Read the model definition and answer for the solid it produces. Units are mm, in the model's axes. Face numbers are marked on the shaded views. A direction names the side the tool comes from. Round coordinates to 2 decimals unless told otherwise and drop trailing zeros. Write each loop counter-clockwise with the first axis right and the second up, starting at its lowest first coordinate (ties: lowest second). Pieces come first, ordered by that corner, then holes. Notation, with made-up numbers: (-13, 5.25) -> (33, 5.25) arc R28 cw to (33, 39.25) -> close; hole circle Ø7 at (45, 9). An arc over 180 degrees is marked (long way). Return JSON: item names as keys, results as strings. Group by question number.
(1) Straight lines are drawn through the part: line 1 (Y direction, x = 3, z = -6.5); line 2 (Y direction, x = -2.5, z = 0); line 3 (X direction, y = 10, z = -9). For each, find the intervals that lie inside material, in ascending order.
(2) Given pin 1 (3 mm diameter, centred on x = 7, y = 17, fed in from -Z); pin 2 (1.5 mm diameter, centred on x = -6.5, y = 23.5, fed in from +Z); pin 3 (3.5 mm diameter, centred on x = -10, y = 15.5, fed in from -Z); pin 4 (1 mm diameter, centred on x = 3.5, z = -15.5, fed in from +Y), each flat-ended and moving along its own axis, determine where each tip first touches the part or whether it passes through.
(3) For the marked faces 4 and 5, determine the directions among +Z, -Z, +X, -X, +Y, -Y from which every point of the face is accessible in a straight line to the end or side of a thin tool.
(4) A cutting plane is placed at A-A on z = 3.5. Give the vertices of the cut face in (x, y), then the cut area to 3 significant figures.
(5) The mould has two halves that part along X. Classify the marked faces 1, 2 and 3: released by +X, released by -X, zero draft, split by the parting line, or undercut.
(6) A cutting plane is placed at C-C on x = 16. Give the vertices of the cut face in (y, z), then the cut area to 3 significant figures.
(7) A cutting plane is placed at D-D on y = 13. Give the vertices of the cut face in (x, z).
(8) A cutting plane is placed at B-B on x = 0. Give the vertices of the cut face in (y, z) (3 decimals), then the cut area to 3 significant figures.
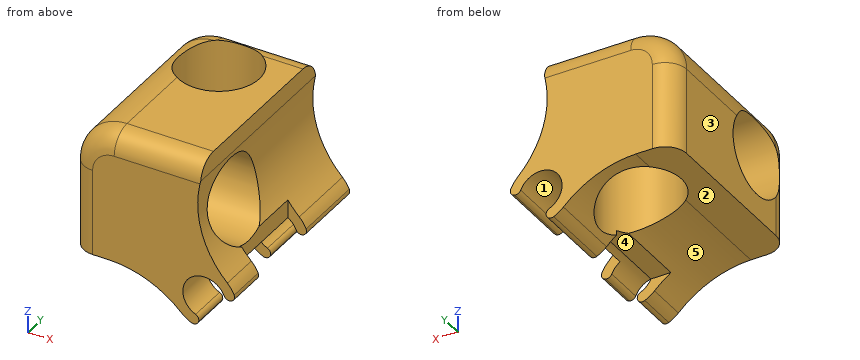
```python
from build123d import *

# Parameters (mm, degrees)
BOSS_EXTRUDE1_DEPTH = 36
SKETCH2_R           = 7.5
CUT_EXTRUDE1_DEPTH  = 51.950145011
SKETCH3_R           = 7.5
CUT_EXTRUDE2_DEPTH  = 52.231763324
FILLET1_R           = 8
FILLET2_R           = 4
FILLET3_R           = 1
FILLET4_R           = 1
CUT_EXTRUDE3_DEPTH  = 7.5


# Some blends are built 0.0001 mm under size
with BuildPart() as part:
    # Sketch1 → Boss-Extrude1 (new body)
    with BuildSketch(Plane(origin=(0, 0, 0), x_dir=(1, 0, 0), z_dir=(0, 1, 0))):
        with BuildLine():
            Line((12.166155414, -12.166155414), (-11.833844586, -12.166155414))
            Line((-11.833844586, -12.166155414), (-11.833844586, 11.833844586))
            Line((-11.833844586, 11.833844586), (-4.753315898, 11.833844586))
            ThreePointArc((-4.753315898, 11.833844586), (2.492071873, 13.348010377), (8.633253511, 17.480107918))
            ThreePointArc((8.633253511, 17.480107918), (9.98514832, 18.495184251), (11.566536194, 19.09285634))
            Line((11.566536194, 19.09285634), (12.002988862, 17.14105997))
            ThreePointArc((12.002988862, 17.14105997), (10.068614763, 10.388049365), (16.792058069, 12.422813601))
            Line((16.792058069, 12.422813601), (18.750140005, 12.015486787))
            ThreePointArc((18.750140005, 12.015486787), (18.154998777, 10.385966776), (17.118534885, 8.994826544))
            ThreePointArc((17.118534885, 8.994826544), (12.32659232, 0.801901017), (12.166155414, -8.688146518))
            Line((12.166155414, -8.688146518), (12.166155414, -12.166155414))
        make_face()
    extrude(amount=BOSS_EXTRUDE1_DEPTH)

    # Sketch2 → Cut-Extrude1 (cut, through all)
    with BuildSketch(Plane.ZY.offset(11.833844586)):
        with Locations((0.166155414, 10)):
            Circle(SKETCH2_R)
    extrude(amount=-CUT_EXTRUDE1_DEPTH, mode=Mode.SUBTRACT)

    # Sketch3 → Cut-Extrude2 (cut, through all)
    with BuildSketch(Plane.XY.offset(12.166155414)):
        with Locations((0.166155414, 26)):
            Circle(SKETCH3_R)
    extrude(amount=-CUT_EXTRUDE2_DEPTH, mode=Mode.SUBTRACT)

    # Fillet1
    # the kernel refuses this fillet: 8 mm, written as the material it takes off along each edge
    with BuildSketch(Plane(origin=(-11.833844586, -20, 12.166155414), x_dir=(1, 0, 0), z_dir=(0, 1, 0))) as fillet1_piece_1:
        with BuildLine():
            CenterArc((FILLET1_R, FILLET1_R), FILLET1_R, 180, 90)
            Line((0, FILLET1_R), (0, 0))
            Line((0, 0), (FILLET1_R, 0))
        make_face()
    extrude(amount=76, mode=Mode.SUBTRACT)

    # Fillet2
    # the kernel refuses this fillet: 4 mm, written as the material it takes off along each edge
    with BuildSketch(Plane(origin=(-11.833844586, 0, 4.166155414), x_dir=(1, 0, 0), z_dir=(0, 0, -1)), Plane(origin=(22.166155414, 36, 12.166155414), x_dir=(0, -1, 0), z_dir=(-1, 0, 0))) as fillet2_piece_1:
        with BuildLine():
            CenterArc((FILLET2_R, -FILLET2_R), FILLET2_R, 90, 90)
            Line((0, -FILLET2_R), (0, 0))
            Line((0, 0), (FILLET2_R, 0))
        make_face()
    extrude(amount=26, mode=Mode.SUBTRACT)
    with BuildSketch(Plane(origin=(-3.833844586, 0, 4.166155414), x_dir=(0, 0, 1), z_dir=(1, 0, 0))) as fillet2_piece_2:
        with BuildLine():
            CenterArc((8 - FILLET2_R, -FILLET2_R), FILLET2_R, 0, 90)
            Line((8, -FILLET2_R), (8, 0))
            Line((8, 0), (8 - FILLET2_R, 0))
        make_face()
    revolve(axis=Axis((-3.833844586, 0, 4.166155414), (0, -1, 0)), revolution_arc=90, mode=Mode.SUBTRACT)
    with BuildSketch(Plane(origin=(-3.833844586, 36, 4.166155414), x_dir=(0, 0, 1), z_dir=(1, 0, 0))) as fillet2_piece_3:
        with BuildLine():
            CenterArc((8 - FILLET2_R, FILLET2_R), FILLET2_R, 270, 90)
            Line((8, FILLET2_R), (8, 0))
            Line((8, 0), (8 - FILLET2_R, 0))
        make_face()
    revolve(axis=Axis((-3.833844586, 36, 4.166155414), (0, -1, 0)), revolution_arc=90, mode=Mode.SUBTRACT)
    with BuildSketch(Plane(origin=(22.166155414, 0, 12.166155414), x_dir=(0, 1, 0), z_dir=(-1, 0, 0)), Plane(origin=(-11.833844586, 36, 4.166155414), x_dir=(1, 0, 0), z_dir=(0, 0, -1))) as fillet2_piece_4:
        with BuildLine():
            CenterArc((FILLET2_R, FILLET2_R), FILLET2_R, 180, 90)
            Line((0, FILLET2_R), (0, 0))
            Line((0, 0), (FILLET2_R, 0))
        make_face()
    extrude(amount=26, mode=Mode.SUBTRACT)

    # Fillet3
    fillet3_edges = [part.edges().sort_by_distance(p)[0] for p in [
        (12.002988862, 18, -17.14105997),
        (16.792058069, 18, -12.422813601),
    ]]
    fillet(fillet3_edges, radius=FILLET3_R)

    # Fillet4
    fillet4_edges = [part.edges().sort_by_distance(p)[0] for p in [
        (11.566536194, 18, -19.09285634),
        (18.750140005, 18, -12.015486787),
    ]]
    fillet(fillet4_edges, radius=FILLET4_R - 0.0001)  # a hair under: the kernel refuses the full size

    # Sketch4 → Cut-Extrude3 (cut, symmetric)
    with BuildSketch(Plane(origin=(0, 15, 0), x_dir=(1, 0, 0), z_dir=(0, 1, 0))):
        Polygon((15, 15), (15, 0), (27.823989989, 3.609418598), (23.424788661, 30.402201484), (6.171676897, 29.445037867), (0, 15), align=None)
    extrude(amount=CUT_EXTRUDE3_DEPTH, both=True, mode=Mode.SUBTRACT)


solid = part.part
```
Checks:
{
 "1": {"line 1": "y = 0 to 6.56, 13.44 to 19.06, 32.94 to 36", "line 2": "y = 0 to 2.5, 17.5 to 18.99, 33.01 to 36", "line 3": "x = -11.83 to 15"},
 "2": {"pin 1": "stops at z = -15", "pin 2": "stops at z = 11.67", "pin 3": "stops at z = -11.83", "pin 4": "passes through"},
 "3": {"face 4": "-Z, +X, -X", "face 5": "-Z, -X, +Y, -Y"},
 "4": {"outline": "(-11.83, 16.72) -> (11.65, 16.72) -> (11.65, 36) -> (-7.83, 36) arc R4 ccw to (-11.83, 32) -> close; (-11.77, 3.28) arc R4 ccw to (-7.83, 0) -> (11.65, 0) -> (11.65, 3.28) -> close; hole circle Ø15 at (0.17, 26)", "area": "346 mm^2"},
 "5": {"face 1": "undercut", "face 2": "zero draft", "face 3": "released by -X"},
 "6": {"outline": "(0, -10.74) -> (7.5, -10.74) -> (7.5, -7.77) -> (0, -7.77) -> close; (22.5, -10.74) -> (36, -10.74) -> (36, -7.77) -> (22.5, -7.77) -> close", "area": "62.3 mm^2"},
 "7": {"outline": "(-11.83, -11.83) -> (-4.75, -11.83) arc R19.28 cw to (5.59, -15) -> (9.29, -15) arc R4 cw to (15, -9.85) -> (15, -6.71) -> (-11.83, -6.71) -> close; (-11.3, 7.04) -> (11.84, 7.04) arc R18.73 cw to (12.17, 8.69) -> (12.17, 12.17) -> (-3.83, 12.17) arc R8 ccw to start"},
 "8": {"outline": "(0, -12.492) -> (18.502, -12.492) -> (18.502, 12.166) -> (4, 12.166) arc R4 ccw to (0, 8.166) -> close; (33.498, -12.492) -> (36, -12.492) -> (36, 8.166) arc R4 ccw to (33.498, 11.875) -> close; hole circle Ø15 at (10, 0.166)", "area": "334 mm^2"}
}
